The drawing under review shows one solid part. Ordinate dimensions are in mm from its lowest x, y, z. A direction names the side the tool comes from. Give positions to 0.01 mm unless a question says otherwise; leave off trailing zeros. Loops run counter-clockwise (first coordinate to the right, second up) from the corner with the lowest first, then second, coordinate; pieces in that order, holes last. Notation, with made-up numbers: (57, 79.25) - (69, 79.25) arc R25 ccw to (69, 98.25) - close; hole circle Ø1 at (7, -36). An arc over 180 degrees is marked (long way). One line per item, written item: value. Start each with the question number.
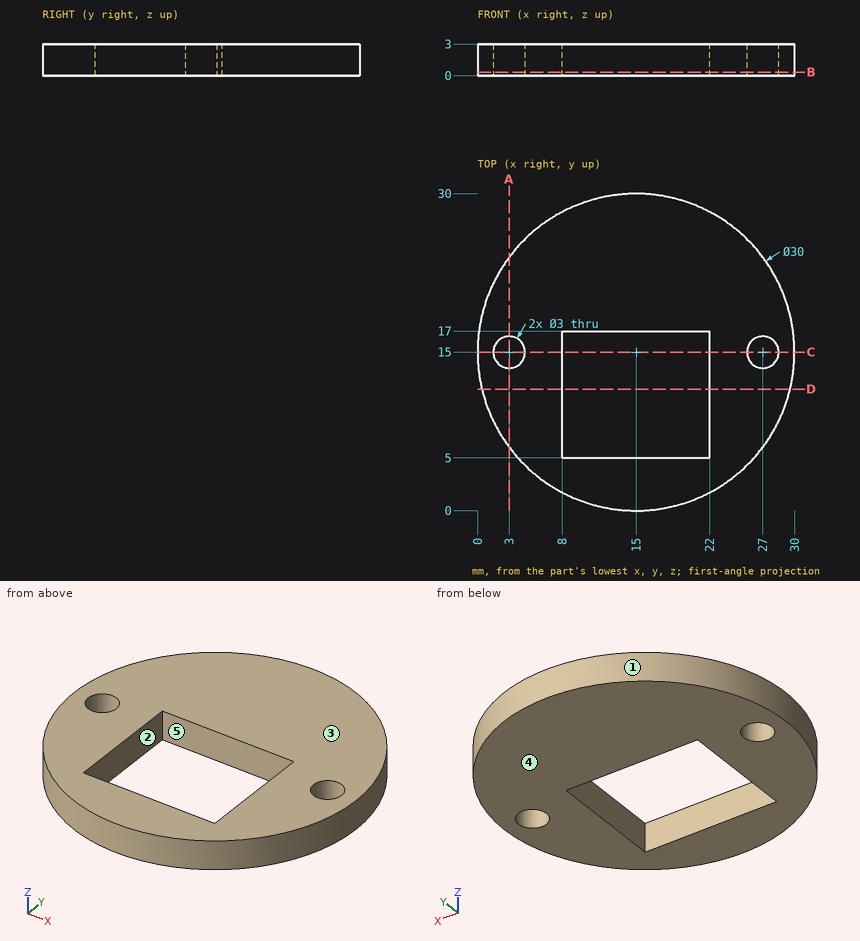
(1) To check wall thickness, follow L1, parallel to Y at x = 15.25, z = 1.4; L2, parallel to X at y = 14, z = 1.7; L3, parallel to Y at x = 27, z = 1. State the ranges of each line that lie inside material, in increasing order. Write a range as from..to.
(2) Take a section at C-C on y = 15. State the section outline as (x, z) points, and give its area (3 significant figures).
(3) Machinability: for the marked faces 4 and 5, which of the approach directions +Z, -Z, +X, -X, +Y, -Y give a long, thin tool a straight path to every point of the face, cutting with its end or side? Answer none if there is none.
(4) Take a section at A-A on x = 3. State the section outline as (y, z) points.
(5) For pin 1 Ø1 at (y, z) = (11, 0.5) entering from -X; pin 2 Ø1 at (y, z) = (24, 1) entering from +X, all flat-tipped, find the tip position at first contact; note any pin that passes through.
(6) Draft analysis for pull direction Y (two halves, no side actions). For the marked faces 1, 2 and 3, state which applies: pulls with the +Y half, pulls with the -Y half, needs draft (parallel to the pull), parting line crosses it, or undercut.
(7) Take a section at D-D on y = 11.5. State the section outline as (x, z) points, and give its area (3 significant figures).
(8) Take a section at B-B on z = 0.35. State the section outline as (x, y) points.
Here are the results:
1. L1: 0..5, 17..30
1. L2: 0.03..1.88, 4.12..8, 22..25.88, 28.12..29.97
1. L3: 6..13.5, 16.5..24
2. outline: (0, 0) - (1.5, 0) - (1.5, 3) - (0, 3) - close; (4.5, 0) - (8, 0) - (8, 3) - (4.5, 3) - close; (22, 0) - (25.5, 0) - (25.5, 3) - (22, 3) - close; (28.5, 0) - (30, 0) - (30, 3) - (28.5, 3) - close
2. area: 30.0 mm²
3. face 4: -Z, +X, -X, +Y, -Y
3. face 5: +Z, -Z
4. outline: (6, 0) - (13.5, 0) - (13.5, 3) - (6, 3) - close; (16.5, 0) - (24, 0) - (24, 3) - (16.5, 3) - close
5. pin 1: x = 0.41
5. pin 2: x = 27.36
6. face 1: parting line crosses it
6. face 2: undercut
6. face 3: needs draft
7. outline: (0.41, 0) - (8, 0) - (8, 3) - (0.41, 3) - close; (22, 0) - (29.59, 0) - (29.59, 3) - (22, 3) - close
7. area: 45.5 mm²
8. outline: circle Ø30 at (15, 15); hole circle Ø3 at (3, 15); hole (8, 5) - (22, 5) - (22, 17) - (8, 17) - close; hole circle Ø3 at (27, 15)
